The model under review builds one solid part; all positions refer to its coordinate system, in mm. Face numbers are marked on the shaded views. A direction names the side the tool comes from. Coordinates: 2 decimals unless noted, no trailing zeros. Loops run counter-clockwise (first coordinate to the right, second up) from the corner with the lowest first, then second, coordinate; pieces in that order, holes last. Notation, with made-up numbers: M 4,23 L 21,23 A27 ccw 21,45 Z; hole C 47.5,63.5 d9. An arc over 180 degrees is marked long. Use CSV: the item, a comma, the result in double quotes. Start each with the question number.
1. Clearance check with flat-ended pins moving along their axes: P1, Ø1, axis at x = 40, y = -5.5, coming from the +Z side; P2, Ø11, axis at y = -22.5, z = 2.5, coming from the +X side; P3, Ø3, axis at x = 47, z = 33.5, coming from the -Y side. State where each tip first meets the part, or that it passes through.
2. Add section A-A, the plane z = 35.5. Write out the cut boundary in (x, y), then the cut area to 3 significant figures.
3. For L1, parallel to Y at x = 22, z = 6; L2, parallel to X at y = -25, z = 9; L3, parallel to Z at x = 29.5, y = -27, list the stretches that pass through material, from the lowest coordinate up.
4. Draft analysis for pull direction Y (two halves, no side actions). For the marked faces 1, 2 and 3, state which applies: +Y half, -Y half, draft (parallel to the pull), parting line (faces both ways), or undercut.
5. Tool access review of the marked faces 4 and 5: name each direction out of +Z, -Z, +X, -X, +Y, -Y from which nothing blocks a thin tool from reaching the whole face with its end or side.
6. Add section C-C, the plane z = 5.5. Write out the cut boundary in (x, y), then the cut area to 3 significant figures.
7. Add section B-B, the plane y = -11.5. Write out the cut boundary in (x, z).
8. Add section D-D, the plane x = 25. Write out the cut boundary in (y, z), then the cut area to 3 significant figures.
from build123d import *

# Parameters (mm, degrees)
F0_W      = 50
F0_H      = 50
F1_DEPTH  = 50
F3_DEPTH  = 43
F5_DEPTH  = 25
F6_DEPTH  = 43
F8_REACH  = 115.9479483752
F12_DEPTH = 35
F13_W     = 20
F13_H     = 10
F14_DEPTH = 30


with BuildPart() as f1:
    # F0 (on Front) → F1 (new body)
    with BuildSketch(Plane.XZ):
        with Locations((25, 25)):
            Rectangle(F0_W, F0_H)
    extrude(amount=F1_DEPTH)

    # F2 (on face) → F3 (cut)
    with BuildSketch(Plane.XY.offset(50)):
        Polygon((15, -50), (50, 0), (35, 0), (0, -50), align=None)
    extrude(amount=-F3_DEPTH, mode=Mode.SUBTRACT)

    # F4 (on face) → F5 (cut)
    with BuildSketch(Plane.XY.offset(50)):
        Polygon((50, -50), (50, -15), (39.5, -15), (15, -50), align=None)
    extrude(amount=-F5_DEPTH, mode=Mode.SUBTRACT)

    # F6 (cut): a face of the model
    f6_faces = [f1.faces().sort_by_distance(p)[0] for p in [
        (11.6666666667, -16.6666666667, 50),
    ]]
    extrude(f6_faces, amount=-F6_DEPTH, mode=Mode.SUBTRACT)

    f8_end = Plane(origin=(36.1029411765, -19.8529411765, 22.3235294118), x_dir=(-0.5734623444, -0.8192319205, 0), z_dir=(-0.8192319205, 0.5734623444, 0))
    # F7 (on face) → F8 (join, up to a plane its end follows)
    with BuildSketch(Plane(origin=(0, 0, 0), x_dir=(0, -1, 0), z_dir=(-1, 0, 0))):
        Polygon((50, 7), (0, 50), (0, 7), align=None)
    f8_long = extrude(amount=-F8_REACH, mode=Mode.PRIVATE)
    add(split(f8_long, bisect_by=f8_end, keep=Keep.TOP, mode=Mode.PRIVATE))

    # F10 (on plane+point) → F12 (cut, through all)
    with BuildSketch(Plane.XY.offset(50)):
        Polygon((15, -50), (50.0000000002, 0), (35.0000000002, 0), (0, -50), align=None)
    extrude(amount=-F12_DEPTH, mode=Mode.SUBTRACT)

    # F13 (on face) → F14 (cut)
    with BuildSketch(Plane.YZ.offset(50)):
        with Locations((-20, 5)):
            Rectangle(F13_W, F13_H)
    extrude(amount=-F14_DEPTH, mode=Mode.SUBTRACT)


solid = f1.part
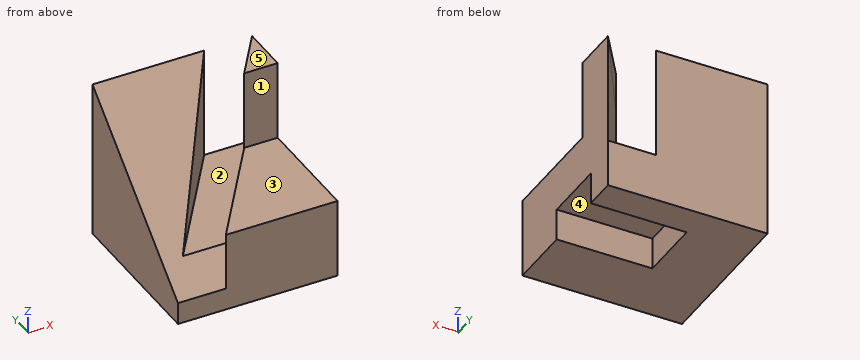
Computed:
1,P1,"stops at z = 15"
1,P2,"stops at x = 20"
1,P3,"stops at y = -15"
2,outline,"M 0,-16.86 L 23.2,-16.86 L 35,0 L 0,0 Z; M 39.5,-15 L 50,-15 L 50,0 Z"
2,area,"569 mm^2"
3,L1,"y = -50 to -30, -10 to 0"
3,L2,"x = 0 to 20"
3,L3,"z = 10 to 15"
4,face 1,"-Y half"
4,face 2,"undercut"
4,face 3,"draft"
5,face 4,"-Z, +X"
5,face 5,"+Z, +X, -X, +Y, -Y"
6,outline,"M 0,-50 L 50,-50 L 50,-30 L 20,-30 L 20,-10 L 50,-10 L 50,0 L 0,0 Z"
6,area,"1,900 mm^2"
7,outline,"M 0,0 L 20,0 L 20,10 L 50,10 L 50,50 L 41.95,50 L 41.95,15 L 26.95,15 L 26.95,40.11 L 0,40.11 Z"
8,outline,"M -50,0 L -30,0 L -30,10 L -10,10 L -10,0 L 0,0 L 0,50 L -14.29,37.71 L -14.29,15 L -35.71,15 L -35.71,25 L -50,25 Z"
8,area,"1,110 mm^2"
